CAD build for the part. Positions are in the model's coordinates, mm. A direction names the side the tool comes from. Round coordinates to 2 decimals unless told otherwise and drop trailing zeros. Loops run counter-clockwise (first coordinate to the right, second up) from the corner with the lowest first, then second, coordinate; pieces in that order, holes last. Notation, with made-up numbers: M 46,30 L 102,30 A17 cw 102,47 Z; hole C 13,-23.75 d10. An arc over 180 degrees is marked long. Use one line per item in the form item = value.
from build123d import *

# Parameters (mm, degrees)
SKETCH1_W           = 80
SKETCH1_H           = 15
BOSS_EXTRUDE1_DEPTH = 3.8


with BuildPart() as part:
    # Sketch1 → Boss-Extrude1 (new body)
    with BuildSketch(Plane(origin=(0, 0, 0), x_dir=(1, 0, 0), z_dir=(0, 1, 0))):
        Rectangle(SKETCH1_W, SKETCH1_H)
        Polygon((-38, 0), (-32.5, -5.5), (-27, 0), (-32.5, 5.5), align=None, mode=Mode.SUBTRACT)
        Polygon((32.5, 5.5), (27, 0), (32.5, -5.5), (38, 0), align=None, mode=Mode.SUBTRACT)
    extrude(amount=BOSS_EXTRUDE1_DEPTH)


solid = part.part
1. Cut at A-A on z = 4. Write the cut outline in (x, y).
Completed:
outline = M -40,0 L -34,0 L -34,3.8 L -40,3.8 Z; M -31,0 L 31,0 L 31,3.8 L -31,3.8 Z; M 34,0 L 40,0 L 40,3.8 L 34,3.8 Z
2. Cut at B-B on y = 1.3. Write the cut outline in (x, z).
Completed:
outline = M -40,-7.5 L 40,-7.5 L 40,7.5 L -40,7.5 Z; hole M -38,0 L -32.5,-5.5 L -27,0 L -32.5,5.5 Z; hole M 27,0 L 32.5,-5.5 L 38,0 L 32.5,5.5 Z
3. Probe line 1 along X through (y, z) = (2, 1.75); line 2 along X through (y, z) = (0.4, 2.5); line 3 along Z through (x, y) = (28, 1.8). List the from-to ranges inside material, lowest first. Write a range as from..to.
Completed:
line_1 = -40..-36.25, -28.75..28.75, 36.25..40
line_2 = -40..-35.5, -29.5..29.5, 35.5..40
line_3 = -7.5..-1, 1..7.5
4. Pull direction Z, two halves, no side cores. Call faces 3 (the face through (30, 2, 3)), 4 (the face through (-40, 2, 0)), 5 (the face through (-1, 2, 7.5)), 6 (the face through (-1, 2, -7.5)): +Z half, -Z half, draft (parallel to the pull), parting line (faces both ways), or undercut.
Completed:
face_3 = undercut
face_4 = draft
face_5 = +Z half
face_6 = -Z half
5. Cut at C-C on z = -2. Write the cut outline in (x, y).
Completed:
outline = M -40,0 L -36,0 L -36,3.8 L -40,3.8 Z; M -29,0 L 29,0 L 29,3.8 L -29,3.8 Z; M 36,0 L 40,0 L 40,3.8 L 36,3.8 Z
6. Tool access for faces 1 (the face through (-30, 2, 3)), 2 (the face through (-1, 3.8, 0)): list every direction of +Z, -Z, +X, -X, +Y, -Y with a clear straight run to the whole face (end or side of a thin tool).
Completed:
face_1 = +Y, -Y
face_2 = +Z, -Z, +X, -X, +Y
